Solid Edge part; units mm, degrees
sketch "Sketch1" plane through (-9.04, 0, 33.0648) normal (0, -1, 0) x (1, 0, 0)
  line L0 (-30.96, -29.0648) -> (5.04, -29.0648)
  line L1 (5.04, -29.0648) -> (5.04, 6.9352)
  line L2 (5.04, 6.9352) -> (9.04, 6.9352)
  line L3 (9.04, 6.9352) -> (9.04, -33.0648)
  line L4 (9.04, -33.0648) -> (-30.96, -33.0648)
  line L5 (-30.96, -33.0648) -> (-30.96, -29.0648)
extrude "Protrusion1" add sketch "Sketch1" along normal mid plane 350
sketch "Sketch2" plane through (-20, 0, 0) normal (0, 0, -1) x (0, -1, 0)
  circle A0 centre (-155, 12) radius 3
  circle A1 centre (-155, -6) radius 3
  dimension "D1" = 155
  dimension "D2" = 155
extrude "Cutout1" cut sketch "Sketch2" against normal through all
mirror "Mirror1" about plane through (0, 0, 0) normal (0, -1, 0) of "Cutout1"
Can you work these out from the model? Positions are in its coordinate system, mm. A direction names the side the tool comes from. Coordinates: 2 decimals unless noted, no trailing zeros. Loops run counter-clockwise (first coordinate to the right, second up) from the corner with the lowest first, then second, coordinate; pieces in that order, holes last.
1) Imagine slicing it at D-D on z = 15.5. List the corners of the cut face in (x, y) for me.
2) Imagine slicing it at B-B on y = 155. List the corners of the cut face in (x, z) for me, plus the area to 3 significant figures.
3) Which directions (+Z, -Z, +X, -X, +Y, -Y) give clear straight access to the entire face, cutting with the end or side of a thin tool? Please do faces 1 (the flat face through (-22, 2, 4)), 2 (the flat face through (-20, 2, 0)).
4) For pin 1 (7 mm diameter, centred on x = -14, y = -155, fed in from +Z); pin 2 (2 mm diameter, centred on y = -73, z = 11, fed in from -X); pin 3 (5.5 mm diameter, centred on x = -32, y = 155, fed in from +Z), each with a flat end and sliding along its axis, tell me the tip position at first contact or that it passes through.
5) Thinking about a two-plate mould opening in Y: for faces 3 (the cylindrical face through (-31.1, -152.14, 1.97)), 4 (the cylindrical face through (-12.85, 152.23, 1.97)), 5 (the flat face through (-4, 2, 22)), 6 (the flat face through (-11, -175, 3.6)), which applies, pulls with the +Y half, pulls with the -Y half, needs draft (parallel to the pull), parting line crosses it, or undercut?
6) Imagine slicing it at C-C on y = 37. List the corners of the cut face in (x, z) for me, plus the area to 3 significant figures.
7) Imagine slicing it at A-A on x = -14. List the corners of the cut face in (y, z) for me.
8) I need wall thicknesses on probe 1 along Y at (x, z) = (-14, 1); probe 2 along X at (y, z) = (-155, 1); probe 3 along Z at (x, y) = (-36, 138). Which ranges of each line are inside material? Lowest first, please.
Completed:
1. outline: (-4, -175) - (0, -175) - (0, 175) - (-4, 175) - close
2. outline: (-40, 0) - (-35, 0) - (-35, 4) - (-40, 4) - close; (-29, 0) - (-17, 0) - (-17, 4) - (-29, 4) - close; (-11, 0) - (0, 0) - (0, 40) - (-4, 40) - (-4, 4) - (-11, 4) - close
2. area: 256 mm2
3. face 1: +Z, -X, +Y, -Y
3. face 2: -Z, +X, -X, +Y, -Y
4. pin 1: stops at z = 4
4. pin 2: stops at x = -4
4. pin 3: passes through
5. face 3: undercut
5. face 4: undercut
5. face 5: needs draft
5. face 6: pulls with the -Y half
6. outline: (-40, 0) - (0, 0) - (0, 40) - (-4, 40) - (-4, 4) - (-40, 4) - close
6. area: 304 mm2
7. outline: (-175, 0) - (-158, 0) - (-158, 4) - (-175, 4) - close; (-152, 0) - (152, 0) - (152, 4) - (-152, 4) - close; (158, 0) - (175, 0) - (175, 4) - (158, 4) - close
8. probe 1: y = -175 to -158, -152 to 152, 158 to 175
8. probe 2: x = -40 to -35, -29 to -17, -11 to 0
8. probe 3: z = 0 to 4
